```python
from build123d import *

# Parameters (mm, degrees)
SKETCH_R        = 25
PAD_DEPTH       = 7
PAD001_DEPTH    = 25
CHAMFER_SIZE    = 15
CHAMFER001_SIZE = 10
FILLET_R        = 2
FILLET001_R     = 2
FILLET002_R     = 2
SKETCH002_R     = 1.5
POCKET_DEPTH    = 35.301
FILLET003_R     = 2
SKETCH003_R     = 1
POCKET001_DEPTH = 32.001
SKETCH004_R     = 3.5
POCKET002_DEPTH = 32.001


with BuildPart() as part:
    # Sketch → Pad (new body)
    with BuildSketch(Plane.XY):
        Circle(SKETCH_R)
    extrude(amount=PAD_DEPTH)

    # Sketch001 → Pad001 (new body)
    with BuildSketch(Plane.XY.offset(7)):
        Polygon((5.3, 21.614464), (10.3, 21.614464), (10.3, 2.5), (24.176399, 2.5), (24.176399, -2.5), (10.3, -2.5), (10.3, -25), (5.3, -25), align=None)
    pad001 = extrude(amount=PAD001_DEPTH)

    # Mirrored: Pad001 across Sketch001 V_Axis
    add(pad001.mirror(Plane(origin=(0, 0, 7), x_dir=(0, 0, 1), z_dir=(1, 0, 0))))

    # Chamfer
    chamfer_edges = [part.edges().sort_by_distance(p)[0] for p in [
        (7.8, 21.614464, 32),
        (-7.8, 21.614464, 32),
    ]]
    chamfer(chamfer_edges, length=CHAMFER_SIZE)

    # Chamfer001
    chamfer001_edges = [part.edges().sort_by_distance(p)[0] for p in [
        (24.176399, 0, 32),
        (-24.176399, 0, 32),
    ]]
    chamfer(chamfer001_edges, length=CHAMFER001_SIZE)

    # Fillet
    fillet_edges = [part.edges().sort_by_distance(p)[0] for p in [
        (10.3, 14.114464, 24.5),
        (10.3, 21.614464, 12),
        (-10.3, 14.114464, 24.5),
        (-10.3, 21.614464, 12),
    ]]
    fillet(fillet_edges, radius=FILLET_R)

    # Fillet001
    fillet001_edges = [part.edges().sort_by_distance(p)[0] for p in [
        (-19.176399, 2.5, 27),
        (-24.176399, 2.5, 14.5),
        (-19.176399, -2.5, 27),
        (-24.176399, -2.5, 14.5),
        (-12.2382, 2.5, 32),
        (-12.2382, -2.5, 32),
    ]]
    fillet(fillet001_edges, radius=FILLET001_R)

    # Fillet002
    fillet002_edges = [part.edges().sort_by_distance(p)[0] for p in [
        (12.2382, 2.5, 32),
        (19.176399, 2.5, 27),
        (24.176399, 2.5, 14.5),
        (24.176399, -2.5, 14.5),
        (19.176399, -2.5, 27),
        (12.2382, -2.5, 32),
    ]]
    fillet(fillet002_edges, radius=FILLET002_R)

    # Sketch002 → Pocket (cut, through all)
    with BuildSketch(Plane.YZ.offset(10.3)):
        with Locations((7.071707, 13.472552)):
            Circle(SKETCH002_R)
        with Locations((-16.31287, 25.611097)):
            Circle(SKETCH002_R)
    extrude(amount=-POCKET_DEPTH, mode=Mode.SUBTRACT)

    # Fillet003
    fillet003_edges = [part.edges().sort_by_distance(p)[0] for p in [
        (-25, 0, 0),
    ]]
    fillet(fillet003_edges, radius=FILLET003_R)

    # Sketch003 → Pocket001 (cut, through all)
    with BuildSketch(Plane(origin=(0, 0, 0), x_dir=(1, 0, 0), z_dir=(0, 0, -1))):
        with Locations((11.667262, 11.667262)):
            Circle(SKETCH003_R)
        with Locations((-11.667262, 11.667262)):
            Circle(SKETCH003_R)
        with Locations((11.667262, -11.667262)):
            Circle(SKETCH003_R)
        with Locations((-11.667262, -11.667262)):
            Circle(SKETCH003_R)
    extrude(amount=-POCKET001_DEPTH, mode=Mode.SUBTRACT)

    # Sketch004 → Pocket002 (cut, through all)
    with BuildSketch(Plane(origin=(0, 0, 0), x_dir=(1, 0, 0), z_dir=(0, 0, -1))):
        Circle(SKETCH004_R)
    extrude(amount=-POCKET002_DEPTH, mode=Mode.SUBTRACT)


solid = part.part
```
Design review of the part built by this model. Coordinates are the model's own, in mm. A direction names the side the tool comes from. Give positions to 0.01 mm unless a question says otherwise; leave off trailing zeros. Order: outer loops, then holes, each group sorted by start corner. A loop starts at its lowest first (then second) coordinate and runs counter-clockwise, first axis right, second up. Notation, with made-up numbers: M 79.5,-31 L 131.5,-31 A33 cw 131.5,5 Z; hole C 49.5,28 d6. An arc over 180 degrees is marked long. One line per question, with ' | ' between items. Start each with the question number.
Q1. We need section C-C (z = 4.5). Write out the cut boundary in (x, y), plus the area to 3 significant figures.
Q2. For L1, parallel to X at y = 0, z = 4; L2, parallel to X at y = 10, z = 14, list the stretches that pass through material, from the lowest coordinate up. Write a range as [from, to].
Q3. We need section A-A (x = 0). Write out the cut boundary in (y, z).
Q4. For pin 1 Ø6 at (x, z) = (14.5, 23.5) entering from -Y; pin 2 Ø2 at (x, z) = (13, 17) entering from +Y; pin 3 Ø4 at (y, z) = (7.07, 13.47) entering from -X; pin 4 Ø1.8 at (y, z) = (-16.31, 25.61) entering from -X, all flat-tipped, find the tip position at first contact; note any pin that passes through.
Q5. The part is to be moulded in two halves that separate along Z. For faces 1 (the face through (-9.73, 12.867, 24.897)), 2 (the face through (-7.76, 5.97, 14.49)), 3 (the face through (8, -24, 7)), say which applies: +Z half, -Z half, draft (parallel to the pull), parting line (faces both ways), or undercut.
Q6. Machinability: for faces 4 (the face through (-23.575, 1.93, 14.605)), 5 (the face through (9.73, 21.01, 12.07)), 6 (the face through (5, 0, 7)), 7 (the face through (-16, -2.5, 16)), which of the approach directions +Z, -Z, +X, -X, +Y, -Y give a long, thin tool a straight path to every point of the face, cutting with its end or side? Answer none if there is none.
Q7. We need section B-B (z = 11). Write out the cut boundary in (x, y).
Returned:
1) outline: C 0,0 d50; hole C -11.67,-11.67 d2; hole C -11.67,11.67 d2; hole C 0,0 d7; hole C 11.67,-11.67 d2; hole C 11.67,11.67 d2 | area: 1,910 mm2
2) L1: [-25, -3.5], [3.5, 25] | L2: [-10.3, -5.3], [5.3, 10.3]
3) outline: M -25,2 A2 ccw -23,0 L -3.5,0 L -3.5,7 L -25,7 Z; M 3.5,0 L 23,0 A2 ccw 25,2 L 25,7 L 3.5,7 Z
4) pin 1: y = -2.5 | pin 2: y = 2.5 | pin 3: x = -10.3 | pin 4: through
5) face 1: +Z half | face 2: undercut | face 3: -Z half
6) face 4: +Z, -X, +Y | face 5: +Z, +X, +Y | face 6: +Z | face 7: +Z, -X, -Y
7) outline: M -24.18,-0.5 A2 ccw -22.18,-2.5 L -10.3,-2.5 L -10.3,-25 L -5.3,-25 L -5.3,21.61 L -8.3,21.61 A2 ccw -10.3,19.61 L -10.3,2.5 L -22.18,2.5 A2 ccw -24.18,0.5 Z; M 5.3,-25 L 10.3,-25 L 10.3,-2.5 L 22.18,-2.5 A2 ccw 24.18,-0.5 L 24.18,0.5 A2 ccw 22.18,2.5 L 10.3,2.5 L 10.3,19.61 A2 ccw 8.3,21.61 L 5.3,21.61 Z
